Autodesk Inventor part; units mm, degrees
ref_plane "Work Plane1" through (66.6877, 0, 0) normal (0, 0, -1) x (1, 0, 0)
ref_plane "YZ Plane" through (0, 0, 0) normal (1, 0, 0) x (0, 1, 0)
ref_plane "XZ Plane" through (0, 0, 0) normal (0, 1, 0) x (-1, 0, 0)
sketch "Szkic1" plane through (0, 0, 0) normal (0, 0, 1) x (1, 0, 0)
  line L0 (4.7625, 0) -> (4.7625, 1.4224)
  line L1 (4.7625, 1.4224) -> (2.1082, 1.4224)
  line L2 (0, 2.7686) -> (0, 0.9144)
  line L3 (0, 0.9144) -> (1.397, 0.9144)
  line L4 (1.397, 0.9144) -> (1.9249, 0)
  line L5 (1.9249, 0) -> (4.7625, 0)
  line L6 (0, 2.7686) -> (0.5596, 2.7686)
  line L7 (0.5596, 2.7686) -> (2.1082, 1.4224)
  line L8 (-0.9525, 0) -> (5.715, 0)
  line L9 (0, -0.5537) -> (0, 3.3223)
  dimension "d0" = 4.7625
  dimension "d1" = 1.397
  dimension "d2" = 2.8448
  dimension "d3" = 2.1082
  dimension "d4" = 41
  dimension "d5" = 1.8288
  dimension "d6" = 60
  dimension "d7" = 5.5372
revolve "Bryła" add sketch "Szkic1" angle 360 about axis through (1.9249, 0, 0) along (1, 0, 0) contours L5 L4 L3 L2 L6 L7 L1 L0
sketch "Szkic2" plane through (0, 0, 0) normal (-1, 0, 0) x (0, 0, 1)
  circle A0 centre (0, 0) radius 2.7686
  circle A1 centre (0, 0) radius 0.9144
  line L0 (0.7066, 0.1893) -> (0.8832, 0.2367)
  line L1 (0.7066, -0.1893) -> (0.8832, -0.2367)
  arc A2 (0.7066, -0.1893) -> (0.7066, 0.1893) centre (0, 0) ccw
  arc A3 (0.8832, -0.2367) -> (0.8832, 0.2367) centre (0, 0) ccw
  line L2 (0, -3.876) -> (0, 3.876)
  line L3 (-3.876, 0) -> (3.876, 0)
  line L4 (0.7066, 0.1893) -> (0, 0) construction
  line L5 (0, 0) -> (0.7066, -0.1893) construction
  line L6 (0.1893, 0.7066) -> (0.2367, 0.8832)
  line L7 (0.5173, 0.5173) -> (0.6466, 0.6466)
  arc A4 (0.5173, 0.5173) -> (0.1893, 0.7066) centre (0, 0) ccw
  arc A5 (0.6466, 0.6466) -> (0.2367, 0.8832) centre (0, 0) ccw
  line L8 (-0.5173, 0.5173) -> (-0.6466, 0.6466)
  line L9 (-0.1893, 0.7066) -> (-0.2367, 0.8832)
  arc A6 (-0.1893, 0.7066) -> (-0.5173, 0.5173) centre (0, 0) ccw
  arc A7 (-0.2367, 0.8832) -> (-0.6466, 0.6466) centre (0, 0) ccw
  line L10 (-0.7066, -0.1893) -> (-0.8832, -0.2367)
  line L11 (-0.7066, 0.1893) -> (-0.8832, 0.2367)
  arc A8 (-0.7066, 0.1893) -> (-0.7066, -0.1893) centre (0, 0) ccw
  arc A9 (-0.8832, 0.2367) -> (-0.8832, -0.2367) centre (0, 0) ccw
  line L12 (-0.1893, -0.7066) -> (-0.2367, -0.8832)
  line L13 (-0.5173, -0.5173) -> (-0.6466, -0.6466)
  arc A10 (-0.5173, -0.5173) -> (-0.1893, -0.7066) centre (0, 0) ccw
  arc A11 (-0.6466, -0.6466) -> (-0.2367, -0.8832) centre (0, 0) ccw
  line L14 (0.5173, -0.5173) -> (0.6466, -0.6466)
  line L15 (0.1893, -0.7066) -> (0.2367, -0.8832)
  arc A12 (0.1893, -0.7066) -> (0.5173, -0.5173) centre (0, 0) ccw
  arc A13 (0.2367, -0.8832) -> (0.6466, -0.6466) centre (0, 0) ccw
  dimension "d8" = 1.463
  dimension "d9" = 1.8288
  dimension "d10" = 15
  dimension "d11" = 15
  dimension "d22" = 360
extrude "Szczelina" add sketch "Szkic2" against normal up to next contours L3 A2 L0 A1 | A1 L1 A2 L3 | L3 A8 L10 A1 | A1 L11 A8 L3 | A1 L7 A4 L6 | L9 A6 L8 A1 | A1 L13 A10 L12 | L15 A12 L14 A1
thread "Gwint"
chamfer "Faza1" distance 0.3175 distance2 0.3175 1 edges at (4.7625, -1.4224, 0) measured on face at (4.7625, -0.1427, 0.3949)
ref_plane "Work Plane1" through (66.6877, 0, 0) normal (0, 0, -1) x (1, 0, 0)
equation "\"d0\" = NLG"
equation "\"d1\" = INTI"
equation "\"d2\" = GD"
equation "\"d3\" = KOH"
equation "\"d4\" = 0.5 * SEWI"
equation "\"d5\" = SW"
equation "\"d7\" = KOD"
equation "\"d8\" = 0.8 * SW"
equation "\"d9\" = SW"
equation "\"d15\" = GEL"
equation "\"d17\" = -0.5 * SPD + 0.5 * GD"
equation "\"d18\" = GUL"
equation "\"NLG\" = 4.7625"
equation "\"SW\" = 1.8288"
equation "\"INTI\" = 1.397"
equation "\"GEL\" = 1.0668"
equation "\"KOH\" = 2.1082"
equation "\"KOD\" = 5.5372"
equation "\"GUL\" = 0.3175"
equation "\"SPD\" = 2.2098"
equation "\"GD\" = NND"
equation "\"SEWI\" = 82deg"
equation "\"TOA\" = 30deg"
equation "\"GD1\" = SPD"
equation "\"EPV\" = 3.80335"
equation "\"THREADDIA\" = 2.8448"
equation "\"BDM\" = NND"
equation "\"NND\" = 2.8448"
equation "\"GAL\" = 1.5875"
equation "\"E0\" = 1.155 * SW"
properties part number "ANSI B18.3 - 4-40 UNC x 0,1875" material "Stal, miękka"
Part model, mm, in its own coordinate system. Give positions to 0.01 mm unless a question says otherwise; leave off trailing zeros. Write each loop counter-clockwise with the first axis right and the second up, starting at its lowest first coordinate (ties: lowest second). Pieces come first, ordered by that corner, then holes.
1) Two-plate mould, pull along Z, no slides. Class faces 1 (the face through (4.762, 0, 0)), 2 (the face through (3.26, -0.31, 1.39)), 3 (the face through (1.89, 0.03, -0.05)): released by +Z, released by -Z, zero draft, split by the parting line, or undercut.
Resolved:
face 1: zero draft
face 2: split by the parting line
face 3: undercut
2) Probe L1, parallel to Z at x = 1.65, y = -0.25; L2, parallel to X at y = -2.45, z = 0.3; L3, parallel to X at y = 1.35, z = 0.2. List the from-to ranges inside material, lowest first.
Resolved:
L1: z = -1.8 to -0.41, 0.41 to 1.8
L2: x = 0 to 0.91
L3: x = 0 to 4.5
3) Cut at A-A on x = 0.3. Write the cut outline in (y, z), then the cut area to 3 significant figures.
Resolved:
outline: circle Ø5.54 at (0, 0); hole (-0.88, -0.24) - (-0.71, -0.19) arc R0.73 ccw to (-0.52, -0.52) - (-0.65, -0.65) arc R0.91 ccw to (-0.24, -0.88) - (-0.19, -0.71) arc R0.73 ccw to (0.19, -0.71) - (0.24, -0.88) arc R0.91 ccw to (0.65, -0.65) - (0.52, -0.52) arc R0.73 ccw to (0.71, -0.19) - (0.88, -0.24) arc R0.91 ccw to (0.88, 0.24) - (0.71, 0.19) arc R0.73 ccw to (0.52, 0.52) - (0.65, 0.65) arc R0.91 ccw to (0.24, 0.88) - (0.19, 0.71) arc R0.73 ccw to (-0.19, 0.71) - (-0.24, 0.88) arc R0.91 ccw to (-0.65, 0.65) - (-0.52, 0.52) arc R0.73 ccw to (-0.71, 0.19) - (-0.88, 0.24) arc R0.91 ccw to start
area: 21.9 mm2
4) Cut at B-B on x = 2.3. Write the cut outline in (y, z), then the cut area to 3 significant figures.
Resolved:
outline: circle Ø2.84 at (0, 0)
area: 6.36 mm2
5) Pin check, flat tip, straight feed: pin 1 (1 mm diameter, centred on x = 4, y = -1.5, fed in from -Z). Stop position of the tip, or through.
Resolved:
pin 1: stops at z = -1.01
6) Cut at C-C on x = 0.8. Write the cut outline in (y, z), then the cut area to 3 significant figures.
Resolved:
outline: circle Ø5.12 at (0, 0); hole (-0.88, -0.24) - (-0.71, -0.19) arc R0.73 ccw to (-0.52, -0.52) - (-0.65, -0.65) arc R0.91 ccw to (-0.24, -0.88) - (-0.19, -0.71) arc R0.73 ccw to (0.19, -0.71) - (0.24, -0.88) arc R0.91 ccw to (0.65, -0.65) - (0.52, -0.52) arc R0.73 ccw to (0.71, -0.19) - (0.88, -0.24) arc R0.91 ccw to (0.88, 0.24) - (0.71, 0.19) arc R0.73 ccw to (0.52, 0.52) - (0.65, 0.65) arc R0.91 ccw to (0.24, 0.88) - (0.19, 0.71) arc R0.73 ccw to (-0.19, 0.71) - (-0.24, 0.88) arc R0.91 ccw to (-0.65, 0.65) - (-0.52, 0.52) arc R0.73 ccw to (-0.71, 0.19) - (-0.88, 0.24) arc R0.91 ccw to start
area: 18.4 mm2
